```python
from build123d import *

# Parameters (mm, degrees)
F0_R     = 2
F1_DEPTH = 5
F2_R     = 15
F3_DEPTH = 4
F5_DEPTH = 5


# Not quite as in the source:
# - after a boolean that leaves OpenCascade's solid faulty, fix() repairs it


with BuildPart() as f1:
    # F0 (on Top) → F1 (new body)
    with BuildSketch(Plane.XY):
        with BuildLine():
            ThreePointArc((0, 28), (-5.3033008589, 25.8033008589), (-7.5, 20.5))
            Line((-7.5, 20.5), (-7.5, 19.5))
            ThreePointArc((-7.5, 19.5), (-11.0147186258, 11.0147186258), (-19.5, 7.5))
            Line((-19.5, 7.5), (-20.5, 7.5))
            ThreePointArc((-20.5, 7.5), (-25.8033008589, 5.3033008589), (-28, 0))
            ThreePointArc((-28, 0), (-25.8033008589, -5.3033008589), (-20.5, -7.5))
            Line((-20.5, -7.5), (-19.5, -7.5))
            ThreePointArc((-19.5, -7.5), (-11.0147186258, -11.0147186258), (-7.5, -19.5))
            Line((-7.5, -19.5), (-7.5, -20.5))
            ThreePointArc((-7.5, -20.5), (-5.3033008589, -25.8033008589), (0, -28))
            ThreePointArc((0, -28), (5.3033008589, -25.8033008589), (7.5, -20.5))
            Line((7.5, -20.5), (7.5, -19.5))
            ThreePointArc((7.5, -19.5), (11.0147186258, -11.0147186258), (19.5, -7.5))
            Line((19.5, -7.5), (20.5, -7.5))
            ThreePointArc((20.5, -7.5), (25.8033008589, -5.3033008589), (28, 0))
            ThreePointArc((28, 0), (25.8033008589, 5.3033008589), (20.5, 7.5))
            Line((20.5, 7.5), (19.5, 7.5))
            ThreePointArc((19.5, 7.5), (11.0147186258, 11.0147186258), (7.5, 19.5))
            Line((7.5, 19.5), (7.5, 20.5))
            ThreePointArc((7.5, 20.5), (5.3033008589, 25.8033008589), (0, 28))
        make_face()
        with Locations((0, -20)):
            Circle(F0_R, mode=Mode.SUBTRACT)
        with Locations((-20, 0)):
            Circle(F0_R, mode=Mode.SUBTRACT)
        with Locations((20, 0)):
            Circle(F0_R, mode=Mode.SUBTRACT)
        with Locations((0, 20)):
            Circle(F0_R, mode=Mode.SUBTRACT)
    extrude(amount=F1_DEPTH)

    # F2 (on Top) → F3 (join)
    with BuildSketch(Plane.XY):
        Circle(F2_R)
    extrude(amount=-F3_DEPTH)

    # F4 (on face) → F5 (join)
    with BuildSketch(Plane(origin=(0, 0, -4), x_dir=(1, 0, 0), z_dir=(0, 0, -1))):
        with BuildLine():
            ThreePointArc((-7.9819098145, 12.6999651855), (-10.6066017178, 10.6066017178), (-12.6999651855, 7.9819098145))
            ThreePointArc((-12.6999651855, 7.9819098145), (-4.6765981284, 4.6765981284), (-7.9819098145, 12.6999651855))
        make_face()
        with BuildLine():
            ThreePointArc((12.6999651855, 7.9819098145), (10.6066017178, 10.6066017178), (7.9819098145, 12.6999651855))
            ThreePointArc((7.9819098145, 12.6999651855), (4.6765981284, 4.6765981284), (12.6999651855, 7.9819098145))
        make_face()
        with BuildLine():
            ThreePointArc((7.9819098145, -12.6999651855), (10.6066017178, -10.6066017178), (12.6999651855, -7.9819098145))
            ThreePointArc((12.6999651855, -7.9819098145), (4.6765981284, -4.6765981284), (7.9819098145, -12.6999651855))
        make_face()
        with BuildLine():
            ThreePointArc((-12.6999651855, -7.9819098145), (-10.6066017178, -10.6066017178), (-7.9819098145, -12.6999651855))
            ThreePointArc((-7.9819098145, -12.6999651855), (-4.6765981284, -4.6765981284), (-12.6999651855, -7.9819098145))
        make_face()
    extrude(amount=F5_DEPTH)

    add(f1.part.fix(), mode=Mode.REPLACE)


solid = f1.part
```
Geometry: final body of the model. Coordinates: model frame, mm. A direction names the side the tool comes from. Coordinates: 2 decimals unless noted, no trailing zeros. Order: outer loops, then holes, each group sorted by start corner. A loop starts at its lowest first (then second) coordinate and runs counter-clockwise, first axis right, second up. Notation, with made-up numbers: (22.5, -31) -> (69.5, -31) arc R34 cw to (69.5, 5) -> close; hole circle Ø10 at (49, 17). An arc over 180 degrees is marked (long way). Write item = value, one per line.
(1) Line query: line 1 (Y direction, x = 0, z = 1.5); line 2 (Y direction, x = -20, z = 1.1); line 3 (X direction, y = -1.5, z = 4). Output: solid intervals per line, ascending.
Solved:
line_1 = -28 to -22, -18 to 18, 22 to 28
line_2 = -7.5 to -2, 2 to 7.5
line_3 = -27.85 to -21.32, -18.68 to 18.68, 21.32 to 27.85
(2) Access query for faces 4 (the cylindrical face through (4.569, -4.788, -6.465)), 5 (the cylindrical face through (0, 28, 2)). Directions: +Z, -Z, +X, -X, +Y, -Y. A direction counts if a zero-diameter tool reaches every point of the face in a straight line with its end or side. Return the directions, or none.
Solved:
face_4 = -Z
face_5 = +Z, -Z, +Y
(3) Cut plane B-B on x = 0. Return loops of the section in (y, z), plus the area to 3 significant figures.
Solved:
outline = (-28, 0) -> (-22, 0) -> (-22, 5) -> (-28, 5) -> close; (-18, 0) -> (-15, 0) -> (-15, -4) -> (15, -4) -> (15, 0) -> (18, 0) -> (18, 5) -> (-18, 5) -> close; (22, 0) -> (28, 0) -> (28, 5) -> (22, 5) -> close
area = 360 mm²
(4) Pull-direction query (X, two-part tool) for faces 1 (the cylindrical face through (-21.6, -1.2, 2.5)), 2 (the flat face through (-8, -8, -9)), 3 (the cylindrical face through (-10.92, 11.11, 2.46)); classes: pulls with the +X half, pulls with the -X half, needs draft (parallel to the pull), parting line crosses it, or undercut.
Solved:
face_1 = undercut
face_2 = needs draft
face_3 = pulls with the -X half
(5) Cut plane D-D on y = 23.5. Return loops of the section in (x, z), plus the area to 3 significant figures.
Solved:
outline = (-6.87, 0) -> (6.87, 0) -> (6.87, 5) -> (-6.87, 5) -> close
area = 68.7 mm²
(6) Pin query (flat end, axial travel): pin 1 Ø0.8 at (y, z) = (-20, 3) entering from +X; pin 2 Ø1.1 at (x, z) = (20, 3) entering from +Y; pin 3 Ø0.8 at (y, z) = (-20, 2) entering from -X; pin 4 Ø3.5 at (x, y) = (0, -20) entering from -Z. Return the tip coordinate at first contact, or that it passes through.
Solved:
pin_1 = 7.5
pin_2 = 7.5
pin_3 = -7.5
pin_4 = through
(7) Cut plane C-C on x = 6.5. Return loops of the section in (y, z).
Solved:
outline = (-24.24, 0) -> (-13.52, 0) -> (-13.52, -4) -> (-12.45, -4) -> (-12.45, -9) -> (-3.55, -9) -> (-3.55, -4) -> (3.55, -4) -> (3.55, -9) -> (12.45, -9) -> (12.45, -4) -> (13.52, -4) -> (13.52, 0) -> (24.24, 0) -> (24.24, 5) -> (-24.24, 5) -> close
(8) Cut plane A-A on z = -5.5. Return loops of the section in (x, y).
Solved:
outline = (-12.7, -7.98) arc R15 ccw to (-7.98, -12.7) arc R4.7 ccw (long way) to start; (-12.7, 7.98) arc R4.7 ccw (long way) to (-7.98, 12.7) arc R15 ccw to start; (7.98, -12.7) arc R15 ccw to (12.7, -7.98) arc R4.7 ccw (long way) to start; (7.98, 12.7) arc R4.7 ccw (long way) to (12.7, 7.98) arc R15 ccw to start
